from build123d import *

# Parameters (mm, degrees)
SKETCH_1_R               = 44.9
SKETCH_1_R_2             = 2.5
SKETCH_1_R_3             = 18.4
EXTRUDE_1_DEPTH          = 16
SKETCH_2_R               = 4
CUT_EXTRUDE_1_DEPTH      = 3
SKETCH_4_R               = 4.5
CUT_EXTRUDE_2_DEPTH      = 5.1
SKETCH_5_R               = 1.5
CUT_EXTRUDE_3_DEPTH      = 10
PATTERN_CIRCULAR_1_COUNT = 12
FILLET_1_R               = 0.5
SKETCH1_R                = 43.15
CUT_EXTRUDE1_DEPTH       = 66.482975056


with BuildPart() as part:
    # 草图1 → 凸台-拉伸1 (new body)
    with BuildSketch(Plane(origin=(0, 0, 0), x_dir=(1, 0, 0), z_dir=(0, 1, 0))):
        with Locations(Location((0, 0, 0), (0, 0, 270))):
            Circle(SKETCH_1_R)
        with Locations(Location((-24.6, 0, 0), (0, 0, 270))):
            Circle(SKETCH_1_R_2, mode=Mode.SUBTRACT)
        with Locations(Location((-12.3, 21.304224933, 0), (0, 0, 270))):
            Circle(SKETCH_1_R_2, mode=Mode.SUBTRACT)
        with Locations(Location((12.3, 21.304224933, 0), (0, 0, 270))):
            Circle(SKETCH_1_R_2, mode=Mode.SUBTRACT)
        with Locations(Location((24.6, 0, 0), (0, 0, 270))):
            Circle(SKETCH_1_R_2, mode=Mode.SUBTRACT)
        with Locations(Location((12.3, -21.304224933, 0), (0, 0, 270))):
            Circle(SKETCH_1_R_2, mode=Mode.SUBTRACT)
        with Locations(Location((-12.3, -21.304224933, 0), (0, 0, 270))):
            Circle(SKETCH_1_R_2, mode=Mode.SUBTRACT)
        with Locations(Location((0, 0, 0), (0, 0, 270))):
            Circle(SKETCH_1_R_3, mode=Mode.SUBTRACT)
    extrude(amount=EXTRUDE_1_DEPTH)

    # 草图2 → 切除-拉伸1 (cut)
    with BuildSketch(Plane.XZ):
        with Locations(Location((-21.304224933, -12.3, 0), (0, 0, 270))):
            Circle(SKETCH_2_R)
        with Locations(Location((0, 24.6, 0), (0, 0, 270))):
            Circle(SKETCH_2_R)
        with Locations(Location((21.304224933, -12.3, 0), (0, 0, 270))):
            Circle(SKETCH_2_R)
    extrude(amount=-CUT_EXTRUDE_1_DEPTH, mode=Mode.SUBTRACT)

    # 草图4 → 切除-拉伸2 (cut)
    with BuildSketch(Plane(origin=(0, 16, 0), x_dir=(1, 0, 0), z_dir=(0, 1, 0))):
        with Locations(Location((-24.6, 0, 0), (0, 0, 270))):
            Circle(SKETCH_4_R)
        with Locations(Location((-12.3, 21.304224933, 0), (0, 0, 270))):
            Circle(SKETCH_4_R)
        with Locations(Location((12.3, 21.304224933, 0), (0, 0, 270))):
            Circle(SKETCH_4_R)
        with Locations(Location((24.6, 0, 0), (0, 0, 270))):
            Circle(SKETCH_4_R)
        with Locations(Location((12.3, -21.304224933, 0), (0, 0, 270))):
            Circle(SKETCH_4_R)
        with Locations(Location((-12.3, -21.304224933, 0), (0, 0, 270))):
            Circle(SKETCH_4_R)
    extrude(amount=-CUT_EXTRUDE_2_DEPTH, mode=Mode.SUBTRACT)

    # 草图5 → 切除-拉伸3 (cut)
    with BuildSketch(Plane(origin=(45, 0, 0), x_dir=(0, 0, -1), z_dir=(1, 0, 0))):
        with Locations((0, 12)):
            Circle(SKETCH_5_R)
    cut_extrude_3 = extrude(amount=-CUT_EXTRUDE_3_DEPTH, mode=Mode.SUBTRACT)

    # 阵列(圆周)1: 切除-拉伸3 ×12 about axis
    pattern_circular_1_axis = Axis((0, 0, 0), (0, 1, 0))
    for i in range(1, PATTERN_CIRCULAR_1_COUNT):
        add(cut_extrude_3.rotate(pattern_circular_1_axis, i * 360 / PATTERN_CIRCULAR_1_COUNT), mode=Mode.SUBTRACT)

    # 圆角1
    fillet_1_edges = [part.edges().sort_by_distance(p)[0] for p in [
        (0, 16, -18.4),
    ]]
    fillet(fillet_1_edges, radius=FILLET_1_R)

    # Sketch1 → Cut-Extrude1 (cut, through all)
    with BuildSketch(Plane(origin=(0, 16, 0), x_dir=(1, 0, 0), z_dir=(0, 1, 0))):
        with Locations(Location((0, 0, 0), (0, 0, 270))):
            Circle(SKETCH1_R)
    extrude(amount=-CUT_EXTRUDE1_DEPTH, mode=Mode.SUBTRACT)


solid = part.part
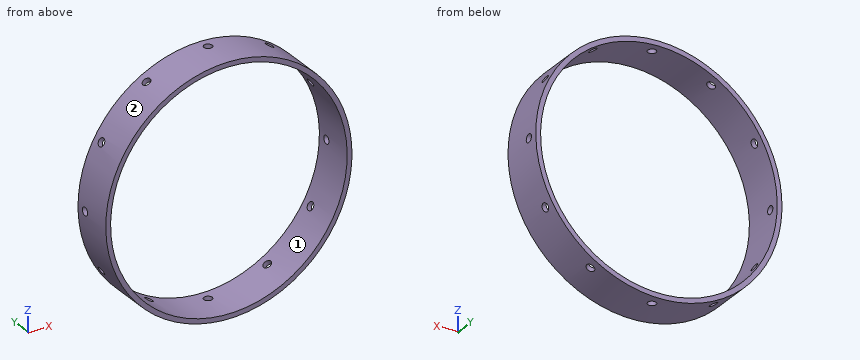
Model file for the job. Use its own axes, mm. Face numbers are marked on the shaded views. Give positions to 0.01 mm unless a question says otherwise; leave off trailing zeros. Write each loop counter-clockwise with the first axis right and the second up, starting at its lowest first coordinate (ties: lowest second). Pieces come first, ordered by that corner, then holes. Notation, with made-up numbers: (28.5, 27) - (46.5, 27) arc R22 ccw to (46.5, 49) - close; hole circle Ø5 at (6.5, 40). An arc over 180 degrees is marked (long way). Answer as CSV lines item,"result".
1. Drill centre lines: L1, parallel to X at y = 5, z = 0; L2, parallel to Z at x = -1, y = 14.25; L3, parallel to Y at x = 0, z = 44.15. Where is each one in solid material? Low to high. Write a range as [from, to].
Responses:
L1,"x = [-44.9, -43.15], [43.15, 44.9]"
L2,"z = [-44.89, -43.14], [43.14, 44.89]"
L3,"y = [0, 10.5], [13.5, 16]"
2. Pin check, flat tips, straight feed: pin 1 (12 mm diameter, centred on x = -30.5, z = -11, fed in from +Y); pin 2 (5 mm diameter, centred on y = 13.5, z = 28.5, fed in from -X); pin 3 (2 mm diameter, centred on y = 11.5, z = -17.5, fed in from +X); pin 4 (5 mm diameter, centred on x = 23.5, y = 9.5, fed in from +Z). Stop position of each tip, or through.
Responses:
pin 1,"passes through"
pin 2,"stops at x = -36.61"
pin 3,"stops at x = 41.76"
pin 4,"stops at z = 39.69"
3. Band-saw the part on D-D (z = -26.5). Write the cut outline in (x, y), and give its area (3 significant figures).
Responses:
outline,"(-36.25, 0) - (-34.05, 0) - (-34.05, 16) - (-36.25, 16) - close; (34.05, 0) - (36.25, 0) - (36.25, 16) - (34.05, 16) - close"
area,"70.1 mm2"
4. Band-saw the part on B-B (x = -25). Write the cut outline in (y, z).
Responses:
outline,"(0, -37.3) - (16, -37.3) - (16, -35.17) - (0, -35.17) - close; (0, 35.17) - (16, 35.17) - (16, 37.3) - (0, 37.3) - close"
5. Two-plate mould, pull along X, no slides. Class the marked faces 1 and 2: +X half, -X half, draft (parallel to the pull), parting line (faces both ways), or undercut.
Responses:
face 1,"undercut"
face 2,"parting line"
6. Band-saw the part on A-A (z = 0). Write the cut outline in (x, y), and give its area (3 significant figures).
Responses:
outline,"(-44.9, 0) - (-43.15, 0) - (-43.15, 10.5) - (-44.9, 10.5) - close; (-44.9, 13.5) - (-43.15, 13.5) - (-43.15, 16) - (-44.9, 16) - close; (43.15, 0) - (44.9, 0) - (44.9, 10.5) - (43.15, 10.5) - close; (43.15, 13.5) - (44.9, 13.5) - (44.9, 16) - (43.15, 16) - close"
area,"45.5 mm2"
7. Band-saw the part on C-C (x = 0). Write the cut outline in (y, z), and give its area (3 significant figures).
Responses:
outline,"(0, -44.9) - (10.5, -44.9) - (10.5, -43.15) - (0, -43.15) - close; (0, 43.15) - (10.5, 43.15) - (10.5, 44.9) - (0, 44.9) - close; (13.5, -44.9) - (16, -44.9) - (16, -43.15) - (13.5, -43.15) - close; (13.5, 43.15) - (16, 43.15) - (16, 44.9) - (13.5, 44.9) - close"
area,"45.5 mm2"
